```python
from build123d import *

# Parameters (mm, degrees)
F1_DEPTH = 152.4
F2_R     = 5.08


with BuildPart() as f1:
    # F0 (on Front) → F1 (new body)
    with BuildSketch(Plane.XZ):
        with BuildLine():
            Line((-9.537221, -24.241146), (1.565489, -24.241146))
            Line((1.565489, -24.241146), (1.56726, -24.209019))
            ThreePointArc((1.56726, -24.209019), (2.697703, -23.759048), (3.168511, -22.637123))
            ThreePointArc((3.168511, -22.637123), (5.764587, -21.304554), (6.538678, -18.490993))
            ThreePointArc((6.538678, -18.490993), (8.729447, -16.190785), (9.526789, -13.11594))
            Line((9.526789, -13.11594), (3.176628, 2.764589))
            Line((3.176628, 2.764589), (3.142439, 2.839835))
            ThreePointArc((3.142439, 2.839835), (5.337396, 3.740061), (6.268152, 5.922246))
            ThreePointArc((6.268152, 5.922246), (5.368231, 8.160809), (3.142439, 9.09187))
            ThreePointArc((3.142439, 9.09187), (2.703335, 10.226903), (1.586881, 10.711301))
            Line((1.586881, 10.711301), (-3.176984, 10.711301))
            Line((-3.176984, 10.711301), (-3.176984, -17.886454))
            Line((-3.176984, -17.886454), (-9.537221, -17.886454))
            Line((-9.537221, -17.886454), (-9.537221, -24.241146))
        make_face()
    extrude(amount=F1_DEPTH)

    # F2
    f2_edges = [f1.edges().sort_by_distance(p)[0] for p in [
        (9.526789, -76.2, -13.11594),
    ]]
    fillet(f2_edges, radius=F2_R)


solid = f1.part
```
Read the model definition and answer for the solid it produces. Units are mm, in the model's axes. A direction names the side the tool comes from. Coordinates: 2 decimals unless noted, no trailing zeros. Write each loop counter-clockwise with the first axis right and the second up, starting at its lowest first coordinate (ties: lowest second). Pieces come first, ordered by that corner, then holes. Notation, with made-up numbers: (-39.75, 82) -> (-29.75, 82) arc R12 ccw to (-29.75, 91) -> close; hole circle Ø4 at (-37.75, 65). An arc over 180 degrees is marked (long way). Return JSON: item names as keys, results as strings.
1. Determine the mould class of faces 1 (the face through (9.364, -77.267, -14.045)), 2 (the face through (0, 0, -10)), 3 (the face through (6.135, -75.133, -4.633)), 4 (the face through (-1, -75, 10.711)) for opening direction Z: pulls with the +Z half, pulls with the -Z half, needs draft (parallel to the pull), parting line crosses it, or undercut.
Found:
{"face 1": "parting line crosses it", "face 2": "needs draft", "face 3": "undercut", "face 4": "pulls with the +Z half"}
2. Find the intervals of material crossed by line 1 along Z through (x, y) = (-8, -53.5); line 2 along X through (y, z) = (-21, 4.5); line 3 along X through (y, z) = (-76, -14), in increasing order. Write a range as from..to.
Found:
{"line 1": "-24.24..-17.89", "line 2": "-3.18..5.9", "line 3": "-3.18..9.37"}
3. A tool of negligible diameter and unlimited length cuts with its end or side. For faces 5 (the face through (0, -152.4, -10)), 6 (the face through (-6, -75, -17.886)), from which of +Z, -Z, +X, -X, +Y, -Y can it reach the whole face along a straight path? Write none if from no direction.
Found:
{"face 5": "+Z, -Z, +X, -X, -Y", "face 6": "+Z, -X, +Y, -Y"}
4. A cutting plane is placed at C-C (z = -4). Determine the outline of the cut face in (x, y), and give its area (3 significant figures).
Found:
{"outline": "(-3.18, -152.4) -> (5.88, -152.4) -> (5.88, 0) -> (-3.18, 0) -> close", "area": "1,380 mm2"}
5. A cutting plane is placed at B-B (x = -6.5). Determine the outline of the cut face in (y, z).
Found:
{"outline": "(-152.4, -24.24) -> (0, -24.24) -> (0, -17.89) -> (-152.4, -17.89) -> close"}
6. Each of these flat-tipped pins is pushed along its axis until it touches: P1, Ø5, axis at x = -7.5, y = -66, coming from the +Z side; P2, Ø3, axis at y = -84.5, z = 0, coming from the -X side; P3, Ø5, axis at y = -134, z = -2, coming from the +X side. Where does it stop, or does it pass through?
Found:
{"P1": "z = -17.89", "P2": "x = -3.18", "P3": "x = 6.08"}
